Can you work these out from the model? Positions are in its coordinate system, mm. A direction names the side the tool comes from. Give positions to 0.01 mm unless a question says otherwise; leave off trailing zeros. Order: outer loops, then holes, each group sorted by start corner. A loop starts at its lowest first (then second) coordinate and runs counter-clockwise, first axis right, second up. Notation, with made-up numbers: (4, 48) - (33, 48) arc R18 ccw to (33, 77) - close; hole circle Ø6 at (6, 21). An arc over 180 degrees is marked (long way). Return JSON: item names as keys, results as strings.
Autodesk Inventor part; units mm, degrees
ref_plane "YZ Plane" through (0, 0, 0) normal (1, 0, 0) x (0, 1, 0)
ref_plane "XZ Plane" through (0, 0, 0) normal (0, 1, 0) x (-1, 0, 0)
ref_plane "XY Plane" through (0, 0, 0) normal (0, 0, 1) x (1, 0, 0)
sketch "スケッチ1" plane through (0, 0, 0) normal (0, 0, 1) x (1, 0, 0)
  circle A0 centre (0, 0) radius 40.5
  circle A1 centre (0, 440) radius 40.5
  line L0 (-40.5, 440) -> (-40.5, 0)
  line L1 (40.5, 0) -> (40.5, 440)
  dimension "d0" = 81
  dimension "d1" = 81
  dimension "d2" = 440
extrude "押し出し1" add sketch "スケッチ1" along normal mid plane 135
sketch "スケッチ2" plane through (0, 0, 0) normal (0, 0, 1) x (1, 0, 0)
  arc A0 (-40.5, 0) -> (40.5, 0) centre (0, 0) ccw
  line L0 (-40.5, 0) -> (-40.5, 440)
  arc A1 (40.5, 440) -> (-40.5, 440) centre (0, 440) ccw
  line L1 (40.5, 440) -> (40.5, 0)
  arc A2 (-40.5, 0) -> (40.5, 0) centre (0, 0) ccw
  line L2 (-40.5, 0) -> (-40.5, 440)
  arc A3 (40.5, 440) -> (-40.5, 440) centre (0, 440) ccw
  line L3 (40.5, 440) -> (40.5, 0)
extrude "押し出し2" cut sketch "スケッチ2" along normal mid plane 84
sketch "スケッチ3" plane through (0, 0, -42) normal (0, 0, 1) x (1, 0, 0)
  circle A0 centre (0, 0) radius 40.5
  point P0 (40.5, 0)
extrude "押し出し3" add sketch "スケッチ3" along normal up to surface (84 mm away)
properties part number "link2"
1. Suppose I cut it at D-D (x = 20.5). List the corners of the cut face in (y, z) for me, plus the area to 3 significant figures.
Checks:
{"outline": "(-34.93, -67.5) - (474.93, -67.5) - (474.93, -42) - (34.93, -42) - (34.93, 42) - (474.93, 42) - (474.93, 67.5) - (-34.93, 67.5) - close", "area": "31,900 mm^2"}
2. On a 3-axis mill with a long thin cutter (end or side, diameter ignored), from which of +Z, -Z, +X, -X, +Y, -Y can I reach the whole of each face in a straight line? I mean faces 1 (the face through (40.5, 217, -55)), 2 (the face through (-5.272, -40.155, -0.945)). Say none if no direction works.
Checks:
{"face 1": "+Z, -Z, +X, +Y, -Y", "face 2": "none"}
3. Suppose I cut it at A-A (y = 305). List the corners of the cut face in (x, z) for me.
Checks:
{"outline": "(-40.5, -67.5) - (40.5, -67.5) - (40.5, -42) - (-40.5, -42) - close; (-40.5, 42) - (40.5, 42) - (40.5, 67.5) - (-40.5, 67.5) - close"}
4. Suppose I cut it at C-C (z = -12.5). List the corners of the cut face in (x, y) for me.
Checks:
{"outline": "circle Ø81 at (0, 0)"}
5. If I drill on L1, parallel to Z at x = -6.5, y = 126.5; L2, parallel to Y at x = -34, z = 59; L3, parallel to Y at x = -30, z = 9, over which ranges is the centre line in solid material (lowest first)? Write a range as [from, to].
Checks:
{"L1": "[-67.5, -42], [42, 67.5]", "L2": "[-22.01, 462.01]", "L3": "[-27.21, 27.21]"}
6. Thinking about a two-plate mould opening in Z: for faces 3 (the face through (-1, 244, -42)), 4 (the face through (40.5, 217, 55)), 5 (the face through (-1, 224, 67.5)), which applies, +Z half, -Z half, draft (parallel to the pull), parting line (faces both ways), or undercut?
Checks:
{"face 3": "undercut", "face 4": "draft", "face 5": "+Z half"}
7. For pin 1 Ø12 at (x, z) = (8, -10.5) entering from +Y; pin 2 Ø1 at (x, z) = (22.5, -50.5) entering from +Y; pin 3 Ø6 at (x, z) = (9, 8.5) entering from +Y, each with a flat end and sliding along its axis, tell me the tip position at first contact or that it passes through.
Checks:
{"pin 1": "y = 40.45", "pin 2": "y = 474", "pin 3": "y = 40.05"}
8. Suppose I cut it at B-B (x = 0). List the corners of the cut face in (y, z) for me, plus the area to 3 significant figures.
Checks:
{"outline": "(-40.5, -67.5) - (480.5, -67.5) - (480.5, -42) - (40.5, -42) - (40.5, 42) - (480.5, 42) - (480.5, 67.5) - (-40.5, 67.5) - close", "area": "33,400 mm^2"}
